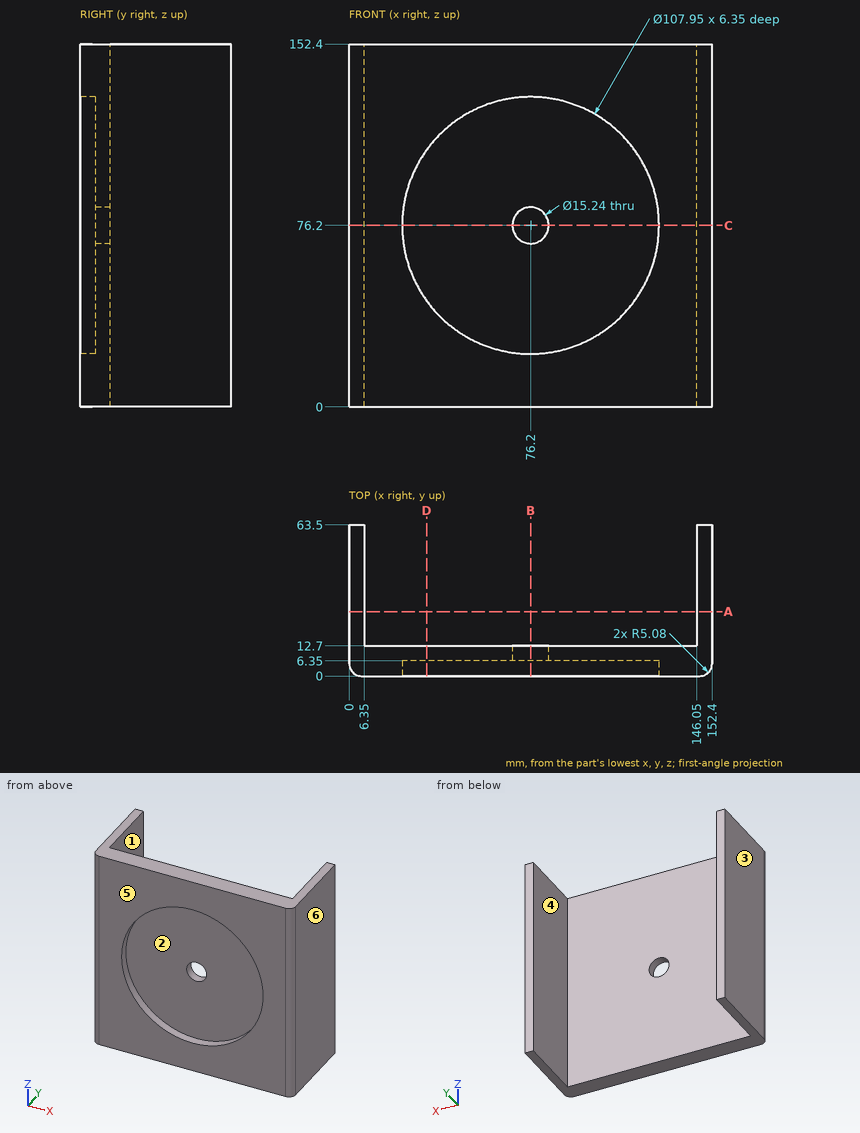
Job drawing, mm, ordinate dimensions from the low corner. One solid piece. A direction names the side the tool comes from. Coordinates: 2 decimals unless noted, no trailing zeros. Order: outer loops, then holes, each group sorted by start corner. A loop starts at its lowest first (then second) coordinate and runs counter-clockwise, first axis right, second up. Notation, with made-up numbers: (33, -30) -> (86, -30) arc R15 cw to (86, -1) -> close; hole circle Ø4 at (80, -3). An arc over 180 degrees is marked (long way). Return JSON: item names as keys, results as strings. Group by question number.
Item 1: Saw through at D-D on x = 32.5. Write the cut outline in (y, z), then the cut area to 3 significant figures.
Item 2: Saw through at A-A on y = 27. Write the cut outline in (x, z), then the cut area to 3 significant figures.
Item 3: Saw through at B-B on x = 76.2. Write the cut outline in (y, z) (3 decimals), then the cut area to 3 significant figures.
Item 4: Pull direction X, two halves, no side cores. Call the marked faces 4, 5 and 6: pulls with the +X half, pulls with the -X half, needs draft (parallel to the pull), parting line crosses it, or undercut.
Item 5: Tool access for the marked faces 1, 2 and 3: list every direction of +Z, -Z, +X, -X, +Y, -Y with a clear straight run to the whole face (end or side of a thin tool).
Item 6: Flat gauge pin, fed straight in: P1, Ø4, axis at x = 42, z = 21.5, coming from the +Y side. Where does the tip first touch, or does it go through?
Item 7: Saw through at C-C on z = 76.2. Write the cut outline in (x, y) (3 decimals), then the cut area to 3 significant figures.
Item 8: Wall check: line 1 along X through (y, z) = (47.5, 20.5); line 2 along Z through (x, y) = (76.2, 5.25) (3 decimals); line 3 along Z through (x, y) = (76.2, 11). Give the ranges that are in metal, low to high. Write a range as [from, to].
Values found:
{
 "1": {"outline": "(0, 0) -> (12.7, 0) -> (12.7, 152.4) -> (0, 152.4) -> (0, 107.88) -> (6.35, 107.88) -> (6.35, 44.52) -> (0, 44.52) -> close", "area": "1,530 mm2"},
 "2": {"outline": "(0, 0) -> (6.35, 0) -> (6.35, 152.4) -> (0, 152.4) -> close; (146.05, 0) -> (152.4, 0) -> (152.4, 152.4) -> (146.05, 152.4) -> close", "area": "1,940 mm2"},
 "3": {"outline": "(0, 0) -> (12.7, 0) -> (12.7, 68.58) -> (6.35, 68.58) -> (6.35, 22.225) -> (0, 22.225) -> close; (0, 130.175) -> (6.35, 130.175) -> (6.35, 83.82) -> (12.7, 83.82) -> (12.7, 152.4) -> (0, 152.4) -> close", "area": "1,150 mm2"},
 "4": {"face 4": "undercut", "face 5": "needs draft", "face 6": "pulls with the +X half"},
 "5": {"face 1": "+Z, -Z, +Y", "face 2": "-Y", "face 3": "+Z, -Z, -X, +Y, -Y"},
 "6": {"P1": "stops at y = 12.7"},
 "7": {"outline": "(0, 5.08) arc R5.08 ccw to (5.08, 0) -> (22.225, 0) -> (22.225, 6.35) -> (68.58, 6.35) -> (68.58, 12.7) -> (6.35, 12.7) -> (6.35, 63.5) -> (0, 63.5) -> close; (83.82, 6.35) -> (130.175, 6.35) -> (130.175, 0) -> (147.32, 0) arc R5.08 ccw to (152.4, 5.08) -> (152.4, 63.5) -> (146.05, 63.5) -> (146.05, 12.7) -> (83.82, 12.7) -> close", "area": "1,790 mm2"},
 "8": {"line 1": "x = [0, 6.35], [146.05, 152.4]", "line 2": "z = [0, 22.225], [130.175, 152.4]", "line 3": "z = [0, 68.58], [83.82, 152.4]"}
}
